The model under review builds one solid part; all positions refer to its coordinate system, in mm. A direction names the side the tool comes from. Round coordinates to 2 decimals unless told otherwise and drop trailing zeros. Order: outer loops, then holes, each group sorted by start corner. A loop starts at its lowest first (then second) coordinate and runs counter-clockwise, first axis right, second up.
from build123d import *

# Parameters (mm, degrees)
SKETCH_2_R          = 2.55
EXTRUDE_1_DEPTH     = 90
SKETCH_3_R          = 3
CUT_EXTRUDE_1_DEPTH = 93.736184955


with BuildPart() as part:
    # 草图2 → 凸台-拉伸1 (new body)
    with BuildSketch(Plane.XY):
        with BuildLine():
            Line((-3.9, 2.839339828), (-6.560660172, 5.5))
            Line((-6.560660172, 5.5), (-8.2, 5.5))
            Line((-8.2, 5.5), (-8.2, 3.1))
            Line((-8.2, 3.1), (-9.45, 3.1))
            Line((-9.45, 3.1), (-9.45, 3.65))
            Line((-9.45, 3.65), (-10, 3.65))
            Line((-10, 3.65), (-10, 8.5))
            ThreePointArc((-10, 8.5), (-9.560660172, 9.560660172), (-8.5, 10))
            Line((-8.5, 10), (-3.65, 10))
            Line((-3.65, 10), (-3.65, 9.45))
            Line((-3.65, 9.45), (-3.1, 9.45))
            Line((-3.1, 9.45), (-3.1, 8.2))
            Line((-3.1, 8.2), (-5.5, 8.2))
            Line((-5.5, 8.2), (-5.5, 6.560660172))
            Line((-5.5, 6.560660172), (-2.839339828, 3.9))
            Line((-2.839339828, 3.9), (2.839339828, 3.9))
            Line((2.839339828, 3.9), (5.5, 6.560660172))
            Line((5.5, 6.560660172), (5.5, 8.2))
            Line((5.5, 8.2), (3.1, 8.2))
            Line((3.1, 8.2), (3.1, 9.45))
            Line((3.1, 9.45), (3.65, 9.45))
            Line((3.65, 9.45), (3.65, 10))
            Line((3.65, 10), (8.5, 10))
            ThreePointArc((8.5, 10), (9.560660172, 9.560660172), (10, 8.5))
            Line((10, 8.5), (10, 3.65))
            Line((10, 3.65), (9.45, 3.65))
            Line((9.45, 3.65), (9.45, 3.1))
            Line((9.45, 3.1), (8.2, 3.1))
            Line((8.2, 3.1), (8.2, 5.5))
            Line((8.2, 5.5), (6.560660172, 5.5))
            Line((6.560660172, 5.5), (3.9, 2.839339828))
            Line((3.9, 2.839339828), (3.9, -2.839339828))
            Line((3.9, -2.839339828), (6.560660172, -5.5))
            Line((6.560660172, -5.5), (8.2, -5.5))
            Line((8.2, -5.5), (8.2, -3.1))
            Line((8.2, -3.1), (9.45, -3.1))
            Line((9.45, -3.1), (9.45, -3.65))
            Line((9.45, -3.65), (10, -3.65))
            Line((10, -3.65), (10, -8.5))
            ThreePointArc((10, -8.5), (9.560660172, -9.560660172), (8.5, -10))
            Line((8.5, -10), (3.65, -10))
            Line((3.65, -10), (3.65, -9.45))
            Line((3.65, -9.45), (3.1, -9.45))
            Line((3.1, -9.45), (3.1, -8.2))
            Line((3.1, -8.2), (5.5, -8.2))
            Line((5.5, -8.2), (5.5, -6.560660172))
            Line((5.5, -6.560660172), (2.839339828, -3.9))
            Line((2.839339828, -3.9), (-2.839339828, -3.9))
            Line((-2.839339828, -3.9), (-5.5, -6.560660172))
            Line((-5.5, -6.560660172), (-5.5, -8.2))
            Line((-5.5, -8.2), (-3.1, -8.2))
            Line((-3.1, -8.2), (-3.1, -9.45))
            Line((-3.1, -9.45), (-3.65, -9.45))
            Line((-3.65, -9.45), (-3.65, -10))
            Line((-3.65, -10), (-8.5, -10))
            ThreePointArc((-8.5, -10), (-9.560660172, -9.560660172), (-10, -8.5))
            Line((-10, -8.5), (-10, -3.65))
            Line((-10, -3.65), (-9.45, -3.65))
            Line((-9.45, -3.65), (-9.45, -3.1))
            Line((-9.45, -3.1), (-8.2, -3.1))
            Line((-8.2, -3.1), (-8.2, -5.5))
            Line((-8.2, -5.5), (-6.560660172, -5.5))
            Line((-6.560660172, -5.5), (-3.9, -2.839339828))
            Line((-3.9, -2.839339828), (-3.9, 2.839339828))
        make_face()
        with Locations(Location((0, 0, 0), (0, 0, 180))):
            Circle(SKETCH_2_R, mode=Mode.SUBTRACT)
    extrude(amount=EXTRUDE_1_DEPTH)

    # 草图3 → 切除-拉伸1 (cut, through all)
    with BuildSketch(Plane(origin=(10, 0, 0), x_dir=(0, 0, -1), z_dir=(1, 0, 0))):
        with Locations(Location((-57.5, 0, 0), (0, 0, 71.16400384))):
            Circle(SKETCH_3_R)
        with Locations((-302.5, 0)):
            Circle(SKETCH_3_R)
    extrude(amount=-CUT_EXTRUDE_1_DEPTH, mode=Mode.SUBTRACT)


solid = part.part
(1) Clearance check with flat-ended pins moving along their axes: P1, Ø4.5, axis at y = 0, z = 72.5, coming from the -X side; P2, Ø0.6, axis at x = -9, z = 28, coming from the +Y side; P3, Ø7, axis at y = 0, z = 57.5, coming from the -X side. State where each tip first meets the part, or that it passes through.
(2) We need section B-B (x = 0). Give the boundary of the cut face in (y, z), and give its area (3 significant figures).
(3) The part is to be moulded in two halves that separate along Y. For faces 1 (the flat face through (7, -5.5, 44)), 2 (the flat face through (5.5, -7, 44)), 3 (the flat face through (-6, 10, 44)), 4 (the flat face through (10, 6, 44)), say which applies: pulls with the +Y half, pulls with the -Y half, needs draft (parallel to the pull), parting line crosses it, or undercut.
(4) Tool access review of faces 5 (the flat face through (-3.9, 0, 28)), 6 (the flat face through (-7, -5.5, 44)), 7 (the flat face through (2, 2, 90)): name each direction out of +Z, -Z, +X, -X, +Y, -Y from which nothing blocks a thin tool from reaching the whole face with its end or side.
(5) To check wall thickness, follow L1, parallel to Y at x = 0, z = 66; L2, parallel to X at y = -8, z = 52.5; L3, parallel to X at y = -4.5, z = 50.5. State the ranges of each line that lie inside material, in increasing order.
(6) We need section A-A (y = 0). Give the boundary of the cut face in (x, z).
Verdict:
1. P1: stops at x = -3.9
1. P2: stops at y = 9.99
1. P3: stops at x = -9.45
2. outline: (-3.9, 0) - (-2.55, 0) - (-2.55, 55.92) arc R3 cw to (-2.55, 59.08) - (-2.55, 90) - (-3.9, 90) - close; (2.55, 0) - (3.9, 0) - (3.9, 90) - (2.55, 90) - (2.55, 59.08) arc R3 cw to (2.55, 55.92) - close
2. area: 241 mm2
3. face 1: undercut
3. face 2: undercut
3. face 3: pulls with the +Y half
3. face 4: needs draft
4. face 5: +Z, -Z, -X
4. face 6: +Z, -Z
4. face 7: +Z, +X, -X, +Y, -Y
5. L1: y = -3.9 to -2.55, 2.55 to 3.9
5. L2: x = -10 to -5.5, 5.5 to 10
5. L3: x = -10 to -8.2, -5.56 to -3.44, 3.44 to 5.56, 8.2 to 10
6. outline: (-3.9, 0) - (-2.55, 0) - (-2.55, 54.5) - (-3.9, 54.5) - close; (-3.9, 60.5) - (-2.55, 60.5) - (-2.55, 90) - (-3.9, 90) - close; (2.55, 0) - (3.9, 0) - (3.9, 54.5) - (2.55, 54.5) - close; (2.55, 60.5) - (3.9, 60.5) - (3.9, 90) - (2.55, 90) - close
